Could you check a few things on this model? Use its own coordinates, in mm. A direction names the side the tool comes from. Round coordinates to 2 decimals unless told otherwise and drop trailing zeros. Order: outer loops, then holes, each group sorted by start corner. A loop starts at its lowest first (then second) coordinate and runs counter-clockwise, first axis right, second up. Notation, with made-up numbers: M 4,33.25 L 63,33.25 A31 ccw 63,72.25 Z; hole C -14.75,62 d5. An arc over 180 degrees is marked long. Write each question's results on one line, items separated by ' | '. Start each with the question number.
1. Please list where these lines run through material, in increasing order: L1, parallel to Y at x = -7.6, z = -0.45; L2, parallel to Y at x = -7.6, z = 1.55; L3, parallel to Z at x = -4, y = -21.5.
2. Suppose I cut it at A-A on z = -0.5. Write out the boundary of the cut face in (x, y).
3. For faces 1 (the cylindrical face through (-14.1, -9.98, -4.09)), 2 (the flat face through (-11, 10.55, -4)), 3 (the flat face through (-8, -23, -2.8)), which set-ups out of +Z, -Z, +X, -X, +Y, -Y let a thin tool reach every point of the face, with its end or its side?
4. We'd pull the mould along Y, two halves only. Please class faces 4 (the flat face through (-19.7, 0, 2)), 5 (the cylindrical face through (-2.885, 25.249, 0.242)), 6 (the flat face through (-12, 6, -8.65)): released by +Y, released by -Y, zero draft, split by the parting line, or undercut.
5. I'm going to push flat-ended pins straight in: pin 1 (5 mm diameter, centred on y = -22, z = 0, fed in from -X); pin 2 (15.5 mm diameter, centred on x = -2.95, y = 0, fed in from -Z); pin 3 (1.1 mm diameter, centred on x = -12, z = -6, fed in from -Y); pin 4 (16 mm diameter, centred on x = -5, y = -3.5, fed in from -Z). Where does each tip first touch, or does it pass through?
6. Suppose I cut it at B-B on y = 0. Write out the boundary of the cut face in (x, z), and give its area (3 significant figures).
7. Suppose I cut it at D-D on x = -7.6. Write out the boundary of the cut face in (y, z).
8. Suppose I cut it at C-C on z = -7.25. Write out the boundary of the cut face in (x, y), and give its area (3 significant figures).
Autodesk Inventor part; units mm, degrees
ref_plane "Work Plane1" through (0, 0, 0.6) normal (0, 0, 1) x (1, 0, 0)
ref_plane "Work Plane2" through (-15.1, -10.95, -8.65) normal (0, 0, 1) x (1, 0, 0)
ref_plane "YZ Plane" through (0, 0, 0) normal (1, 0, 0) x (0, 1, 0)
ref_plane "Work Plane1" through (0, 0, 0.6) normal (0, 0, 1) x (1, 0, 0)
sketch "Sketch1" plane through (0, 0, 0.6) normal (0, 0, 1) x (1, 0, 0)
  circle A0 centre (-11.825, -7.675) radius 1.2
  circle A1 centre (-11.825, 7.675) radius 1.2
  line L0 (-14.7, 10.55) -> (-8.95, 10.55)
  line L1 (-8.95, 10.55) -> (-8.95, 4.8)
  line L2 (-8.95, 4.8) -> (-14.7, 4.8)
  line L3 (-14.7, 4.8) -> (-14.7, 10.55)
  line L4 (-14.7, 10.55) -> (-8.95, 4.8) construction
  line L5 (-8.95, 10.55) -> (-14.7, 4.8) construction
  line L6 (-14.7, -10.55) -> (-8.95, -10.55)
  line L7 (-8.95, -10.55) -> (-8.95, -4.8)
  line L8 (-8.95, -4.8) -> (-14.7, -4.8)
  line L9 (-14.7, -4.8) -> (-14.7, -10.55)
  line L10 (-14.7, -10.55) -> (-8.95, -4.8) construction
  line L11 (-8.95, -10.55) -> (-14.7, -4.8) construction
  arc A2 (-19.7, -8.45) -> (-12.6, -15.55) centre (-12.6, -8.45) ccw
  line L12 (-12.6, -15.55) -> (12.6, -15.55)
  arc A3 (12.6, -15.55) -> (19.7, -8.45) centre (12.6, -8.45) ccw
  line L13 (19.7, -8.45) -> (19.7, -7)
  line L14 (19.7, -7) -> (15.7, -7)
  line L15 (15.7, -7) -> (15.7, -8.45)
  arc A4 (12.6, -11.55) -> (15.7, -8.45) centre (12.6, -8.45) ccw
  line L16 (12.6, -11.55) -> (-12.6, -11.55)
  arc A5 (-15.7, -8.45) -> (-12.6, -11.55) centre (-12.6, -8.45) ccw
  line L17 (-15.7, -8.45) -> (-15.7, 8.45)
  arc A6 (-12.6, 11.55) -> (-15.7, 8.45) centre (-12.6, 8.45) ccw
  line L18 (-12.6, 11.55) -> (12.6, 11.55)
  arc A7 (15.7, 8.45) -> (12.6, 11.55) centre (12.6, 8.45) ccw
  line L19 (15.7, 8.45) -> (15.7, 7)
  line L20 (15.7, 7) -> (19.7, 7)
  line L21 (19.7, 7) -> (19.7, 8.45)
  arc A8 (19.7, 8.45) -> (12.6, 15.55) centre (12.6, 8.45) ccw
  line L22 (12.6, 15.55) -> (-12.6, 15.55)
  arc A9 (-12.6, 15.55) -> (-19.7, 8.45) centre (-12.6, 8.45) ccw
  line L23 (-19.7, 8.45) -> (-19.7, -8.45)
  point P0 (0, 0)
  dimension "d1" = 1
  dimension "d2" = 1
ref_plane "Work Plane2" through (-15.1, -10.95, -8.65) normal (0, 0, 1) x (1, 0, 0)
extrude "Extrusion1" add sketch "Sketch1" against normal up to surface (9.25 mm away) contours A0 | A1 | L0 L1 L2 L3 | L9 L8 L7 L6
fillet "Fillet1" radius 2 4 edges at (-14.7, 10.55, -4.025) (-14.7, -10.55, -4.025) (-8.95, 4.8, -4.025) (-8.95, -4.8, -4.025)
sketch "Sketch2" plane through (-10.95, 4.8, -8.65) normal (0, 0, -1) x (-1, 0, 0)
  circle A0 centre (0.875, 2.875) radius 1.2
  circle A1 centre (0.875, -12.475) radius 1.2
  point P0 (-10.95, -4.8)
extrude "Extrusion2" add sketch "Sketch2" along normal blind 3
chamfer "Chamfer1" distance 0.6 angle 45 2 edges at (-10.625, 7.675, -11.65) (-10.625, -7.675, -11.65)
sketch "Sketch3" plane through (0, 0, 0.6) normal (0, 0, 1) x (1, 0, 0)
  arc A0 (-19.7, -8.45) -> (-12.6, -15.55) centre (-12.6, -8.45) ccw
  line L0 (-12.6, -15.55) -> (12.6, -15.55)
  arc A1 (12.6, -15.55) -> (19.7, -8.45) centre (12.6, -8.45) ccw
  line L1 (19.7, -8.45) -> (19.7, -7)
  line L2 (19.7, -7) -> (15.7, -7)
  line L3 (15.7, -7) -> (15.7, -8.45)
  arc A2 (12.6, -11.55) -> (15.7, -8.45) centre (12.6, -8.45) ccw
  line L4 (12.6, -11.55) -> (-12.6, -11.55)
  arc A3 (-15.7, -8.45) -> (-12.6, -11.55) centre (-12.6, -8.45) ccw
  line L5 (-15.7, -8.45) -> (-15.7, 8.45)
  arc A4 (-12.6, 11.55) -> (-15.7, 8.45) centre (-12.6, 8.45) ccw
  line L6 (-12.6, 11.55) -> (12.6, 11.55)
  arc A5 (15.7, 8.45) -> (12.6, 11.55) centre (12.6, 8.45) ccw
  line L7 (15.7, 8.45) -> (15.7, 7)
  line L8 (15.7, 7) -> (19.7, 7)
  line L9 (19.7, 7) -> (19.7, 8.45)
  arc A6 (19.7, 8.45) -> (12.6, 15.55) centre (12.6, 8.45) ccw
  line L10 (12.6, 15.55) -> (-12.6, 15.55)
  arc A7 (-12.6, 15.55) -> (-19.7, 8.45) centre (-12.6, 8.45) ccw
  line L11 (-19.7, 8.45) -> (-19.7, -8.45)
  circle A8 centre (-11.825, 7.675) radius 1.2
  circle A9 centre (-11.825, -7.675) radius 1.2
  line L12 (19.7, 7) -> (15.7, 7)
  line L13 (15.7, 7) -> (15.7, 8.45)
  arc A10 (15.7, 8.45) -> (12.6, 11.55) centre (12.6, 8.45) ccw
  line L14 (12.6, 11.55) -> (-12.6, 11.55)
  arc A11 (-12.6, 11.55) -> (-15.7, 8.45) centre (-12.6, 8.45) ccw
  line L15 (-15.7, 8.45) -> (-15.7, -8.45)
  arc A12 (-15.7, -8.45) -> (-12.6, -11.55) centre (-12.6, -8.45) ccw
  line L16 (-12.6, -11.55) -> (12.6, -11.55)
  arc A13 (12.6, -11.55) -> (15.7, -8.45) centre (12.6, -8.45) ccw
  line L17 (15.7, -8.45) -> (15.7, -7)
  line L18 (15.7, -7) -> (19.7, -7)
  line L19 (19.7, 7) -> (19.7, -7)
  line L20 (15.7, -7) -> (15.7, 7)
  point P0 (0, 0)
extrude "Extrusion3" add sketch "Sketch3" along normal blind 2.6 contours L11 A7 L10 A6 L9 L8 L7 A5 L6 A4 L5 A3 L4 A2 L3 L2 L1 A1 L0 A0 | L2 L20 L8 L19 | L3 A2 L4 A3 L5 A4 L6 A5 L7 L20 | A8 | A9
sketch "Sketch4" plane through (0, 0, 3.2) normal (0, 0, 1) x (1, 0, 0)
  circle A0 centre (-2.95, 0) radius 5.7
  circle A1 centre (-2.95, 0) radius 6.7
  point P0 (0, 0)
  dimension "d13" = 1
extrude "Extrusion4" cut sketch "Sketch4" against normal through all contours A0 | A1
sketch "Sketch5" plane through (0, 0, 3.2) normal (0, 0, 1) x (1, 0, 0)
  circle A0 centre (-2.95, 0) radius 6.7
  line L0 (19.7, -8.45) -> (19.7, 8.45)
  arc A1 (19.7, 8.45) -> (12.6, 15.55) centre (12.6, 8.45) ccw
  line L1 (12.6, 15.55) -> (-12.6, 15.55)
  arc A2 (-12.6, 15.55) -> (-19.7, 8.45) centre (-12.6, 8.45) ccw
  line L2 (-19.7, 8.45) -> (-19.7, -8.45)
  arc A3 (-19.7, -8.45) -> (-12.6, -15.55) centre (-12.6, -8.45) ccw
  line L3 (-12.6, -15.55) -> (12.6, -15.55)
  arc A4 (12.6, -15.55) -> (19.7, -8.45) centre (12.6, -8.45) ccw
  arc A5 (-12.6, -24.55) -> (-11.6, -25.55) centre (-11.6, -24.55) ccw
  line L4 (-11.6, -25.55) -> (-3.6, -25.55)
  arc A6 (-3.6, -25.55) -> (-2.6, -24.55) centre (-3.6, -24.55) ccw
  line L5 (-2.6, -24.55) -> (-2.6, -16.55)
  arc A7 (-1.6, -15.55) -> (-2.6, -16.55) centre (-1.6, -16.55) ccw
  line L6 (-1.6, -15.55) -> (-12.6, -15.55)
  arc A8 (-13.4765, -15.4957) -> (-12.6, -15.55) centre (-12.6, -8.45) ccw
  arc A9 (-12.6, -16.488) -> (-13.4765, -15.4957) centre (-13.6, -16.488) ccw
  line L7 (-12.6, -16.488) -> (-12.6, -24.55)
  circle A10 centre (-7.6, -20.55) radius 2.25
  arc A11 (-2.6, 24.55) -> (-3.6, 25.55) centre (-3.6, 24.55) ccw
  line L8 (-3.6, 25.55) -> (-11.6, 25.55)
  arc A12 (-11.6, 25.55) -> (-12.6, 24.55) centre (-11.6, 24.55) ccw
  line L9 (-12.6, 24.55) -> (-12.6, 16.488)
  arc A13 (-13.4765, 15.4957) -> (-12.6, 16.488) centre (-13.6, 16.488) ccw
  arc A14 (-12.6, 15.55) -> (-13.4765, 15.4957) centre (-12.6, 8.45) ccw
  line L10 (-1.6, 15.55) -> (-12.6, 15.55)
  arc A15 (-2.6, 16.55) -> (-1.6, 15.55) centre (-1.6, 16.55) ccw
  line L11 (-2.6, 16.55) -> (-2.6, 24.55)
  circle A16 centre (-7.6, 20.55) radius 2.25
  line L12 (-12.6, -16.488) -> (-12.6, -15.55)
  line L13 (-2.6, -16.55) -> (-2.6, -15.55)
  line L14 (-12.6, 16.488) -> (-12.6, 15.55)
  line L15 (-2.6, 16.55) -> (-2.6, 15.55)
  point P0 (0, 0)
extrude "Extrusion5" add sketch "Sketch5" against normal blind 6 contours L13 L5 A6 L4 A5 L7 L12 L3 | L1 L14 L9 A12 L8 A11 L11 L15
sketch "Sketch6" plane through (-12.6, 15.55, 0.6) normal (0, -1, 0) x (1, 0, 0)
  line L0 (10, 0) -> (0, 0)
  line L1 (0, 0) -> (0, -3.4)
  line L2 (10, -3.4) -> (0, -3.4)
  line L3 (10, 0) -> (10, -3.4)
  point P0 (12.6, -0.6)
extrude "Extrusion6" cut sketch "Sketch6" against normal blind 0.6
mirror "Mirror1" about plane through (0, 0, 0) normal (0, 1, 0) of "Extrusion6"
equation "\"d2\" = d1"
properties part number "PrzyciskSTOP_2_3DPrint"
Filled sheet:
1) L1: y = -25.55 to -22.8, -18.3 to -16.15, 16.15 to 18.3, 22.8 to 25.55 | L2: y = -25.55 to -22.8, -18.3 to -4.82, 4.82 to 18.3, 22.8 to 25.55 | L3: z = -2.8 to 3.2
2) outline: M -14.7,-8.55 A2 ccw -12.7,-10.55 L -8.95,-10.55 L -8.95,-6.8 A2 ccw -10.95,-4.8 L -14.7,-4.8 Z; M -14.7,4.8 L -10.95,4.8 A2 ccw -8.95,6.8 L -8.95,10.55 L -12.7,10.55 A2 ccw -14.7,8.55 Z; M -12.6,-24.55 A1 ccw -11.6,-25.55 L -3.6,-25.55 A1 ccw -2.6,-24.55 L -2.6,-16.15 L -12.6,-16.15 Z; M -12.6,16.15 L -2.6,16.15 L -2.6,24.55 A1 ccw -3.6,25.55 L -11.6,25.55 A1 ccw -12.6,24.55 Z; hole C -7.6,-20.55 d4.5; hole C -7.6,20.55 d4.5
3) face 1: -Z, -X, -Y | face 2: -Z, +X, -X | face 3: -Z, +X, -X, -Y
4) face 4: zero draft | face 5: released by +Y | face 6: undercut
5) pin 1: stops at x = -12.6 | pin 2: stops at z = 0.6 | pin 3: stops at y = -10.55 | pin 4: stops at z = -11.65
6) outline: M -19.7,0.6 L -9.65,0.6 L -9.65,3.2 L -19.7,3.2 Z; M 3.75,0.6 L 19.7,0.6 L 19.7,3.2 L 3.75,3.2 Z | area: 67.6 mm^2
7) outline: M -25.55,-2.8 L -22.8,-2.8 L -22.8,3.2 L -25.55,3.2 Z; M -18.3,-2.8 L -16.15,-2.8 L -16.15,0.6 L -4.82,0.6 L -4.82,3.2 L -18.3,3.2 Z; M 4.82,0.6 L 16.15,0.6 L 16.15,-2.8 L 18.3,-2.8 L 18.3,3.2 L 4.82,3.2 Z; M 22.8,-2.8 L 25.55,-2.8 L 25.55,3.2 L 22.8,3.2 Z
8) outline: M -14.7,-8.55 A2 ccw -12.7,-10.55 L -8.95,-10.55 L -8.95,-6.8 A2 ccw -10.95,-4.8 L -14.7,-4.8 Z; M -14.7,4.8 L -10.95,4.8 A2 ccw -8.95,6.8 L -8.95,10.55 L -12.7,10.55 A2 ccw -14.7,8.55 Z | area: 62.7 mm^2
